Verification items for the finished model (mm, model axes). A direction names the side the tool comes from. Round coordinates to 2 decimals unless told otherwise and drop trailing zeros. Order: outer loops, then holes, each group sorted by start corner. A loop starts at its lowest first (then second) coordinate and runs counter-clockwise, first axis right, second up. Notation, with made-up numbers: M 22,7.5 L 43,7.5 A20 ccw 43,41.5 Z; hole C 64,43.5 d9. An arc over 180 degrees is marked long. Use one line per item in the form item = value. Start each with the question number.
Item 1: Cross-section at A-A on x = -9. Enter the section's corners in (y, z).
Item 2: Cross-section at D-D on z = -0.7. Enter the section's corners in (x, y), then the cut area to 3 significant figures.
Item 3: Tool access check on faces 1 (the flat face through (-10, 2, -3.162)), 2 (the flat face through (-1, 2, -2.062)), 3 (the flat face through (-13.004, 2, -3)), 4 (the flat face through (-8, 2, 0.338)). Record the directions out of +Z, -Z, +X, -X, +Y, -Y that give a thin tool (end or side, any length) a straight path to the whole face; none if there is none.
Item 4: Cross-section at B-B on x = -11.5. Enter the section's corners in (y, z), then the cut area to 3 significant figures.
Item 5: Go/stop test with flat-tipped pins: pin 1 Ø2 at (x, z) = (-5, -2.5) entering from +Y; pin 2 Ø0.6 at (y, z) = (1.5, 0) entering from -X; pin 3 Ø0.6 at (y, z) = (2, -2.5) entering from -X; pin 4 Ø1.1 at (y, z) = (2, -3.5) entering from +X. Record where each tip stops, or that it passes through.
Item 6: Cross-section at C-C on y = 3.4. Enter the section's corners in (x, z), then the cut area to 3 significant figures.
Item 7: Release check for a two-part mould opening along Z. For faces 5 (the flat face through (-8, 2, -0.862)), 6 (the flat face through (-11, 2, -4.162)), 7 (the flat face through (-2.204, 2, 0)), 8 (the flat face through (-6.504, 2, -3)) record: +Z half, -Z half, draft (parallel to the pull), parting line (faces both ways), or undercut.
Item 8: Thickness scan on probe 1 along Z at (x, y) = (-9.5, 3.25); probe 2 along Z at (x, y) = (-5.5, 2.7); probe 3 along Z at (x, y) = (-0.5, 1.3). Record the ranges inside material, lowest first. Write a range as [from, to].
from build123d import *

# Parameters (mm, degrees)
BOSS_EXTRUDE1_DEPTH = 5
FILLET1_R           = 1


with BuildPart() as part:
    # Sketch1 → Boss-Extrude1 (new body)
    with BuildSketch(Plane(origin=(0, 0, 0), x_dir=(1, 0, 0), z_dir=(0, 1, 0))):
        Polygon((-8.753636364, 4.161818182), (-6.503636364, 4.161818182), (-6.503636364, 2.061818182), (3.796363636, 2.061818182), (3.796363636, -1.538181818), (-14.503636364, -1.538181818), (-14.503636364, -0.338181818), (-2.203636364, -0.338181818), (-2.203636364, 0.861818182), (-14.503636364, 0.861818182), (-14.503636364, 2.061818182), (-13.003636364, 2.061818182), (-13.003636364, 4.161818182), (-10.753636364, 4.161818182), (-10.753636364, 3.161818182), (-8.753636364, 3.161818182), align=None)
    extrude(amount=BOSS_EXTRUDE1_DEPTH)

    # Fillet1
    fillet1_edges = [part.edges().sort_by_distance(p)[0] for p in [
        (-13.003636364, 2.5, -4.161818182),
        (-6.503636364, 2.5, -4.161818182),
    ]]
    fillet(fillet1_edges, radius=FILLET1_R)


solid = part.part
Output values:
q1.outline = M 0,-3.16 L 5,-3.16 L 5,-0.86 L 0,-0.86 Z; M 0,0.34 L 5,0.34 L 5,1.54 L 0,1.54 Z
q2.outline = M -2.2,0 L 3.8,0 L 3.8,5 L -2.2,5 Z
q2.area = 30.0 mm2
q3.face_1 = -Z, +Y, -Y
q3.face_2 = -Z, +X, +Y, -Y
q3.face_3 = -Z, -X, +Y, -Y
q3.face_4 = -X, +Y, -Y
q4.outline = M 0,-4.16 L 5,-4.16 L 5,-0.86 L 0,-0.86 Z; M 0,0.34 L 5,0.34 L 5,1.54 L 0,1.54 Z
q4.area = 22.5 mm2
q5.pin_1 = 5
q5.pin_2 = -2.2
q5.pin_3 = -13
q5.pin_4 = -6.5
q6.outline = M -14.5,-2.06 L -13,-2.06 L -13,-3.16 A1 ccw -12,-4.16 L -10.75,-4.16 L -10.75,-3.16 L -8.75,-3.16 L -8.75,-4.16 L -7.5,-4.16 A1 ccw -6.5,-3.16 L -6.5,-2.06 L 3.8,-2.06 L 3.8,1.54 L -14.5,1.54 L -14.5,0.34 L -2.2,0.34 L -2.2,-0.86 L -14.5,-0.86 Z
q6.area = 62.3 mm2
q7.face_5 = undercut
q7.face_6 = -Z half
q7.face_7 = undercut
q7.face_8 = draft
q8.probe_1 = [-3.16, -0.86], [0.34, 1.54]
q8.probe_2 = [-2.06, -0.86], [0.34, 1.54]
q8.probe_3 = [-2.06, 1.54]
